from build123d import *

# Parameters (mm, degrees)
SKETCH_2_R       = 15
SKETCH_2_R_2     = 6.5
SKETCH_2_R_3     = 1.5
EXTRUDE_1_DEPTH  = 2
CHAMFER_1_SIZE   = 2
CHAMFER_1_SIZE_2 = 1.93137755
SKETCH_3_R       = 1
EXTRUDE_2_DEPTH  = 2


with BuildPart() as part:
    # 草图2 → 凸台-拉伸1 (new body)
    with BuildSketch(Plane(origin=(0, 0, 0), x_dir=(1, 0, 0), z_dir=(0, 1, 0))):
        with Locations(Location((0, 0, 0), (0, 0, 270))):
            Circle(SKETCH_2_R)
        with Locations(Location((0, 0, 0), (0, 0, 270))):
            Circle(SKETCH_2_R_2, mode=Mode.SUBTRACT)
        with Locations(Location((9.5, 0, 0), (0, 0, 270))):
            Circle(SKETCH_2_R_3, mode=Mode.SUBTRACT)
        with Locations(Location((-4.75, -8.227241336, 0), (0, 0, 270))):
            Circle(SKETCH_2_R_3, mode=Mode.SUBTRACT)
        with Locations(Location((-4.75, 8.227241336, 0), (0, 0, 270))):
            Circle(SKETCH_2_R_3, mode=Mode.SUBTRACT)
    extrude(amount=EXTRUDE_1_DEPTH)

    # 倒角1
    # the kernel refuses this chamfer: 2, 1.93137755 mm, written as the material it takes off along each edge
    with BuildSketch(Plane(origin=(-4.75, 0, 8.227241336), x_dir=(0, 0, 1), z_dir=(-1, 0, 0))) as chamfer_1_piece_1:
        Polygon((1.5, CHAMFER_1_SIZE), (1.5 + CHAMFER_1_SIZE_2, 0), (1.5, 0), align=None)
    revolve(axis=Axis((-4.75, 0, 8.227241336), (0, 1, 0)), mode=Mode.SUBTRACT)
    with BuildSketch(Plane(origin=(-4.75, 0, -8.227241336), x_dir=(0, 0, 1), z_dir=(-1, 0, 0))) as chamfer_1_piece_2:
        Polygon((1.5, CHAMFER_1_SIZE), (1.5 + CHAMFER_1_SIZE_2, 0), (1.5, 0), align=None)
    revolve(axis=Axis((-4.75, 0, -8.227241336), (0, 1, 0)), mode=Mode.SUBTRACT)
    with BuildSketch(Plane(origin=(9.5, 0, 0), x_dir=(0, 0, 1), z_dir=(-1, 0, 0))) as chamfer_1_piece_3:
        Polygon((1.5, CHAMFER_1_SIZE), (1.5 + CHAMFER_1_SIZE_2, 0), (1.5, 0), align=None)
    revolve(axis=Axis((9.5, 0, 0), (0, 1, 0)), mode=Mode.SUBTRACT)

    # 草图3 → 凸台-拉伸2 (add)
    # profile 1 of 4: a face of its own
    with BuildSketch(Plane(origin=(0, 0, 0), x_dir=(1, 0, 0), z_dir=(0, 1, 0))):
        with BuildLine():
            Line((-18.5, -3.5), (-14.585952146, -3.5))
            ThreePointArc((-14.585952146, -3.5), (-15, 0), (-14.585952146, 3.5))
            Line((-14.585952146, 3.5), (-18.5, 3.5))
            ThreePointArc((-18.5, 3.5), (-22, 0), (-18.5, -3.5))
        make_face()
        with Locations(Location((-18.5, 0, 0), (0, 0, 270))):
            Circle(SKETCH_3_R, mode=Mode.SUBTRACT)
    # profile 2 of 4: a face of its own
    with BuildSketch(Plane(origin=(0, 0, 0), x_dir=(1, 0, 0), z_dir=(0, 1, 0))):
        with BuildLine():
            Line((-3.5, 18.5), (-3.5, 14.585952146))
            ThreePointArc((-3.5, 14.585952146), (0, 15), (3.5, 14.585952146))
            Line((3.5, 14.585952146), (3.5, 18.5))
            ThreePointArc((3.5, 18.5), (0, 22), (-3.5, 18.5))
        make_face()
        with Locations(Location((0, 18.5, 0), (0, 0, 270))):
            Circle(SKETCH_3_R, mode=Mode.SUBTRACT)
    # profile 3 of 4: a face of its own
    with BuildSketch(Plane(origin=(0, 0, 0), x_dir=(1, 0, 0), z_dir=(0, 1, 0))):
        with BuildLine():
            Line((18.5, 3.5), (14.585952146, 3.5))
            ThreePointArc((14.585952146, 3.5), (15, 0), (14.585952146, -3.5))
            Line((14.585952146, -3.5), (18.5, -3.5))
            ThreePointArc((18.5, -3.5), (22, 0), (18.5, 3.5))
        make_face()
        with Locations(Location((18.5, 0, 0), (0, 0, 270))):
            Circle(SKETCH_3_R, mode=Mode.SUBTRACT)
    # profile 4 of 4: a face of its own
    with BuildSketch(Plane(origin=(0, 0, 0), x_dir=(1, 0, 0), z_dir=(0, 1, 0))):
        with BuildLine():
            Line((3.5, -18.5), (3.5, -14.585952146))
            ThreePointArc((3.5, -14.585952146), (0, -15), (-3.5, -14.585952146))
            Line((-3.5, -14.585952146), (-3.5, -18.5))
            ThreePointArc((-3.5, -18.5), (0, -22), (3.5, -18.5))
        make_face()
        with Locations(Location((0, -18.5, 0), (0, 0, 270))):
            Circle(SKETCH_3_R, mode=Mode.SUBTRACT)
    extrude(amount=EXTRUDE_2_DEPTH)


solid = part.part
Can you work these out from the model? Positions are in its coordinate system, mm. A direction names the side the tool comes from. Coordinates: 2 decimals unless noted, no trailing zeros. Write each loop counter-clockwise with the first axis right and the second up, starting at its lowest first coordinate (ties: lowest second). Pieces come first, ordered by that corner, then holes. Notation, with made-up numbers: (14.5, 74) - (62.5, 74) arc R27 ccw to (62.5, 109) - close; hole circle Ø8 at (87.5, 29). An arc over 180 degrees is marked (long way). Return JSON: item names as keys, results as strings. Group by question number.
Item 1: If we section it at C-C (z = 0): Write out the boundary of the cut face in (x, y).
Item 2: If we section it at A-A (x = 0): Write out the boundary of the cut face in (y, z).
Item 3: If we section it at B-B (y = 0.7): Count the separate pieces of the cut face and the enclosed holes in it, then the cut area to 3 significant figures.
Item 4: We'd pull the mould along Z, two halves only. Please class faces 1 (the face through (-17, 1, -3.5)), 2 (the face through (-19.476, 0.986, -0.217)), 3 (the face through (3.5, 1, 17)), 4 (the face through (-3.955, 0.986, -5.158)): pulls with the +Z half, pulls with the -Z half, needs draft (parallel to the pull), parting line crosses it, or undercut.
Item 5: Which directions (+Z, -Z, +X, -X, +Y, -Y) give clear straight access to the entire face, cutting with the end or side of a thin tool? Please do faces 5 (the face through (3.5, 1, -17)), 6 (the face through (-3.5, 1, 17)), 7 (the face through (-7, 0, 2)).
Item 6: Please list where these lines run through material, in increasing order: probe 1 along X at (y, z) = (1.2, 18.5); probe 2 along X at (y, z) = (0.65, 0); probe 3 along Z at (x, y) = (-4, 0.95).
Item 7: If we section it at D-D (x = 9.5): Write out the boundary of the cut face in (y, z), then the cut area to 3 significant figures.
Item 8: I'm going to push flat-ended pins straight in: pin 1 Ø2.5 at (x, z) = (0, -18.5) entering from +Y; pin 2 Ø0.6 at (x, y) = (-17, 1) entering from -Z; pin 3 Ø0.6 at (x, y) = (-17, 1.5) entering from +Z; pin 4 Ø1 at (y, z) = (1.5, -16.5) entering from -X. Where does each tip first touch, or does it pass through?
Return value:
{
 "1": {"outline": "(-22, 0) - (-19.5, 0) - (-19.5, 2) - (-22, 2) - close; (-17.5, 0) - (-6.5, 0) - (-6.5, 2) - (-17.5, 2) - close; (6.5, 0.45) - (8, 2) - (6.5, 2) - close; (11, 2) - (12.93, 0) - (17.5, 0) - (17.5, 2) - close; (19.5, 0) - (22, 0) - (22, 2) - (19.5, 2) - close"},
 "2": {"outline": "(0, -22) - (2, -22) - (2, -19.5) - (0, -19.5) - close; (0, -17.5) - (2, -17.5) - (2, -6.5) - (0, -6.5) - close; (0, 6.5) - (2, 6.5) - (2, 17.5) - (0, 17.5) - close; (0, 19.5) - (2, 19.5) - (2, 22) - (0, 22) - close"},
 "3": {"separate pieces": "1", "enclosed holes": "8", "area": "669 mm^2"},
 "4": {"face 1": "pulls with the -Z half", "face 2": "undercut", "face 3": "needs draft", "face 4": "undercut"},
 "5": {"face 5": "-Z, +X, +Y, -Y", "face 6": "+Z, -X, +Y, -Y", "face 7": "+Z, -Z, +X, -X, -Y"},
 "6": {"probe 1": "x = -3.5 to -1, 1 to 3.5", "probe 2": "x = -22 to -19.5, -17.5 to -6.5, 6.5 to 6.7, 12.3 to 17.5, 19.5 to 22", "probe 3": "z = -14.46 to -10.63, -5.83 to -5.12, 5.12 to 5.83, 10.63 to 14.46"},
 "7": {"outline": "(0, -11.61) - (2, -11.61) - (2, -1.5) - (0, -3.43) - close; (0, 3.43) - (2, 1.5) - (2, 11.61) - (0, 11.61) - close", "area": "36.6 mm^2"},
 "8": {"pin 1": "stops at y = 2", "pin 2": "stops at z = -3.5", "pin 3": "stops at z = 3.5", "pin 4": "stops at x = -3.5"}
}
